```python
from build123d import *

# Parameters (mm, degrees)
SKETCH1_W           = 72
SKETCH1_H           = 72
BOSS_EXTRUDE1_DEPTH = 5
HOLE1_D             = 62.6
HOLE1_DEPTH         = 2.25
SKETCH4_W           = 27.8
SKETCH4_H           = 2.25
HOLE2_D             = 6.5
HOLE3_D             = 52
CHAMFER1_SIZE       = 2
FILLET1_R           = 5


with BuildPart() as part:
    # Sketch1 → Boss-Extrude1 (new body)
    with BuildSketch(Plane(origin=(0, 0, 0), x_dir=(-1, 0, 0), z_dir=(0, 0, -1))):
        with Locations((-36, 36)):
            Rectangle(SKETCH1_W, SKETCH1_H)
    extrude(amount=-BOSS_EXTRUDE1_DEPTH)

    # Hole1
    with Locations(Plane(origin=(0, 0, 0), x_dir=(-1, 0, 0), z_dir=(0, 0, -1))):
        with Locations((-36, 36)):
            Hole(HOLE1_D / 2, depth=HOLE1_DEPTH)

    # Sketch4 → Revolve1 (revolve)
    with BuildSketch(Plane(origin=(0, 36, 0), x_dir=(1, 0, 0), z_dir=(0, 1, 0)), mode=Mode.PRIVATE) as revolve1_sk:
        with Locations((49.9, -1.125)):
            Rectangle(SKETCH4_W, SKETCH4_H)
    revolve(revolve1_sk.sketch.rotate(Axis((36, 36, 0), (0, 0, 1)), 180), axis=Axis((36, 36, 0), (0, 0, 1)))

    # Hole2 (through all)
    with Locations(Plane.XY.offset(5)):
        with Locations((66, 6), (6, 6), (6, 66), (66, 66)):
            Hole(HOLE2_D / 2)

    # Hole3 (through all)
    with Locations(Plane.XY.offset(5)):
        with Locations((36, 36)):
            Hole(HOLE3_D / 2)

    # Chamfer1
    chamfer1_edges = [part.edges().sort_by_distance(p)[0] for p in [
        (62, 36, 5),
    ]]
    chamfer(chamfer1_edges, length=CHAMFER1_SIZE)

    # Fillet1
    fillet1_edges = [part.edges().sort_by_distance(p)[0] for p in [
        (72, 0, 2.5),
        (72, 72, 2.5),
        (0, 72, 2.5),
        (0, 0, 2.5),
    ]]
    fillet(fillet1_edges, radius=FILLET1_R)


solid = part.part
```
Could you check a few things on this model? Use its own coordinates, in mm. A direction names the side the tool comes from. Round coordinates to 2 decimals unless told otherwise and drop trailing zeros. Loops run counter-clockwise (first coordinate to the right, second up) from the corner with the lowest first, then second, coordinate; pieces in that order, holes last. Notation, with made-up numbers: (-21, 33) -> (-5, 33) arc R18 cw to (-5, 56) -> close; hole circle Ø4 at (59, 40.25). An arc over 180 degrees is marked (long way). Put each result on its own line as item: value.
Q1. I want a section at B-B on x = 36. Write out the boundary of the cut face in (y, z).
Checks:
outline: (0, 0) -> (4.7, 0) -> (4.7, 2.25) -> (8.2, 2.25) -> (8.2, 0) -> (10, 0) -> (10, 3) -> (8, 5) -> (0, 5) -> close; (62, 0) -> (63.8, 0) -> (63.8, 2.25) -> (67.3, 2.25) -> (67.3, 0) -> (72, 0) -> (72, 5) -> (64, 5) -> (62, 3) -> close
Q2. Thinking about a two-plate mould opening in X: for faces 3 (the flat face through (72, 36, 2)), 4 (the flat face through (36, 0, 2)), 5 (the cylindrical face through (64.913, 24.012, 1.141)), which applies, pulls with the +X half, pulls with the -X half, needs draft (parallel to the pull), parting line crosses it, or undercut?
Checks:
face 3: pulls with the +X half
face 4: needs draft
face 5: undercut
Q3. For pin 1 Ø7.5 at (x, y) = (6, 6) entering from -Z; pin 2 Ø6 at (x, y) = (6, 66) entering from +Z, each with a flat end and sliding along its axis, tell me the tip position at first contact or that it passes through.
Checks:
pin 1: z = 0
pin 2: through
Q4. I want a section at C-C on y = 6. Write out the boundary of the cut face in (x, z), and give its area (3 significant figures).
Checks:
outline: (0, 0) -> (2.75, 0) -> (2.75, 5) -> (0, 5) -> close; (9.25, 0) -> (27.07, 0) -> (27.07, 2.25) -> (44.93, 2.25) -> (44.93, 0) -> (62.75, 0) -> (62.75, 5) -> (9.25, 5) -> close; (69.25, 0) -> (72, 0) -> (72, 5) -> (69.25, 5) -> close
area: 255 mm2
Q5. Which directions (+Z, -Z, +X, -X, +Y, -Y) give clear straight access to the entire face, cutting with the end or side of a thin tool? Please do faces 1 (the flat face through (37, 69, 0)), 2 (the flat face through (36, 64, 2.25)).
Checks:
face 1: -Z, +X, -X, +Y, -Y
face 2: -Z
Q6. Please list where these lines run through material, in increasing order: line 1 (Y direction, x = 36, z = 1.5); line 2 (X direction, y = 29.5, z = 2.1). Write a range as from..to.
Checks:
line 1: 0..4.7, 8.2..10, 62..63.8, 67.3..72
line 2: 0..5.38, 8.97..10.83, 61.17..63.03, 66.62..72
Q7. I want a section at A-A on z = 0.85. Write out the boundary of the cut face in (x, y), and give its area (3 significant figures).
Checks:
outline: (0, 5) arc R5 ccw to (5, 0) -> (67, 0) arc R5 ccw to (72, 5) -> (72, 67) arc R5 ccw to (67, 72) -> (5, 72) arc R5 ccw to (0, 67) -> close; circle Ø55.6 at (36, 36); hole circle Ø6.5 at (6, 6); hole circle Ø6.5 at (6, 66); hole circle Ø62.6 at (36, 36); hole circle Ø52 at (36, 36); hole circle Ø6.5 at (66, 6); hole circle Ø6.5 at (66, 66)
area: 2,260 mm2
